Work out the finished part from the listing and answer in its coordinate system (mm). Face numbers are marked on the shaded views. Round coordinates to 2 decimals unless told otherwise and drop trailing zeros. Loops run counter-clockwise (first coordinate to the right, second up) from the corner with the lowest first, then second, coordinate; pieces in that order, holes last.
```python
from build123d import *

# Parameters (mm, degrees)
BOSS_EXTRUDE1_DEPTH = 36
SKETCH2_R           = 4.25
CUT_EXTRUDE1_DEPTH  = 32.7
SKETCH3_W           = 36
SKETCH3_H           = 0.5
CUT_EXTRUDE2_DEPTH  = 72.2


with BuildPart() as part:
    # Sketch1 → Boss-Extrude1 (new body)
    with BuildSketch(Plane.XY):
        with BuildLine():
            Line((-73.529829319, 33.051903281), (-144.729829319, 33.051903281))
            Line((-144.729829319, 33.051903281), (-144.729829319, 1.351903281))
            Line((-144.729829319, 1.351903281), (-125.829829319, 1.351903281))
            ThreePointArc((-125.829829319, 1.351903281), (-109.129829319, 18.051903281), (-92.429829319, 1.351903281))
            Line((-92.429829319, 1.351903281), (-73.529829319, 1.351903281))
            Line((-73.529829319, 1.351903281), (-73.529829319, 33.051903281))
        make_face()
    extrude(amount=BOSS_EXTRUDE1_DEPTH)

    # Sketch2 → Cut-Extrude1 (cut, through all)
    with BuildSketch(Plane(origin=(0, 33.051903281, 0), x_dir=(1, 0, 0), z_dir=(0, 1, 0))):
        with Locations((-82.628590119, -18)):
            Circle(SKETCH2_R)
        with Locations((-135.631068518, -18)):
            Circle(SKETCH2_R)
    extrude(amount=-CUT_EXTRUDE1_DEPTH, mode=Mode.SUBTRACT)

    # Sketch3 → Cut-Extrude2 (cut, through all)
    with BuildSketch(Plane.ZY.offset(144.729829319)):
        with Locations((18, 1.601903281)):
            Rectangle(SKETCH3_W, SKETCH3_H)
    extrude(amount=-CUT_EXTRUDE2_DEPTH, mode=Mode.SUBTRACT)


solid = part.part
```
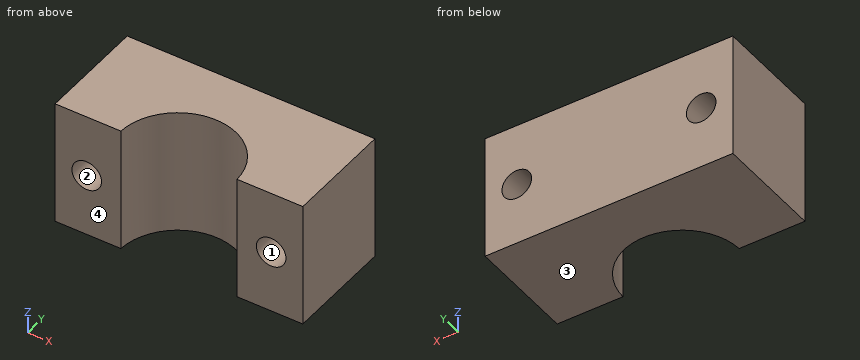
1. Find section C-C (y = 19.5). Write down the section's boundary in (x, z), then the cut area to 3 significant figures.
Answer key:
outline: (-144.73, 0) - (-73.53, 0) - (-73.53, 36) - (-144.73, 36) - close; hole circle Ø8.5 at (-135.63, 18); hole circle Ø8.5 at (-82.63, 18)
area: 2,450 mm2
2. Determine the mould class of the marked faces 1, 2, 3 and 4 for opening direction Z: +Z half, -Z half, draft (parallel to the pull), parting line (faces both ways), or undercut.
Answer key:
face 1: undercut
face 2: undercut
face 3: -Z half
face 4: draft
3. Given pin 1 (7 mm diameter, centred on x = -82.63, z = 18, fed in from +Y); pin 2 (1.5 mm diameter, centred on x = -115.5, z = 16.5, fed in from -Y), each flat-ended and moving along its own axis, determine where each tip first touches the part or whether it passes through.
Answer key:
pin 1: passes through
pin 2: stops at y = 16.46
4. Consider probe 1 along X at (y, z) = (20, 18); probe 2 along X at (y, z) = (13, 18); probe 3 along X at (y, z) = (18.5, 16). Determine where each line is inside the solid, lowest interval first.
Answer key:
probe 1: x = -144.73 to -139.88, -131.38 to -86.88, -78.38 to -73.53
probe 2: x = -144.73 to -139.88, -131.38 to -121.1, -97.16 to -86.88, -78.38 to -73.53
probe 3: x = -144.73 to -139.38, -131.88 to -86.38, -78.88 to -73.53
5. Find section B-B (y = 8.5). Write down the section's boundary in (x, z), then the cut area to 3 significant figures.
Answer key:
outline: (-144.73, 0) - (-124.22, 0) - (-124.22, 36) - (-144.73, 36) - close; (-94.04, 0) - (-73.53, 0) - (-73.53, 36) - (-94.04, 36) - close; hole circle Ø8.5 at (-135.63, 18); hole circle Ø8.5 at (-82.63, 18)
area: 1,360 mm2
6. Find section D-D (x = -139). Write down the section's boundary in (y, z).
Answer key:
outline: (1.85, 0) - (33.05, 0) - (33.05, 15.41) - (1.85, 15.41) - close; (1.85, 20.59) - (33.05, 20.59) - (33.05, 36) - (1.85, 36) - close
7. Find section A-A (z = 18). Write down the section's boundary in (x, y), then the cut area to 3 significant figures.
Answer key:
outline: (-144.73, 1.85) - (-139.88, 1.85) - (-139.88, 33.05) - (-144.73, 33.05) - close; (-131.38, 1.85) - (-125.82, 1.85) arc R16.7 cw to (-92.44, 1.85) - (-86.88, 1.85) - (-86.88, 33.05) - (-131.38, 33.05) - close; (-78.38, 1.85) - (-73.53, 1.85) - (-73.53, 33.05) - (-78.38, 33.05) - close
area: 1,270 mm2
